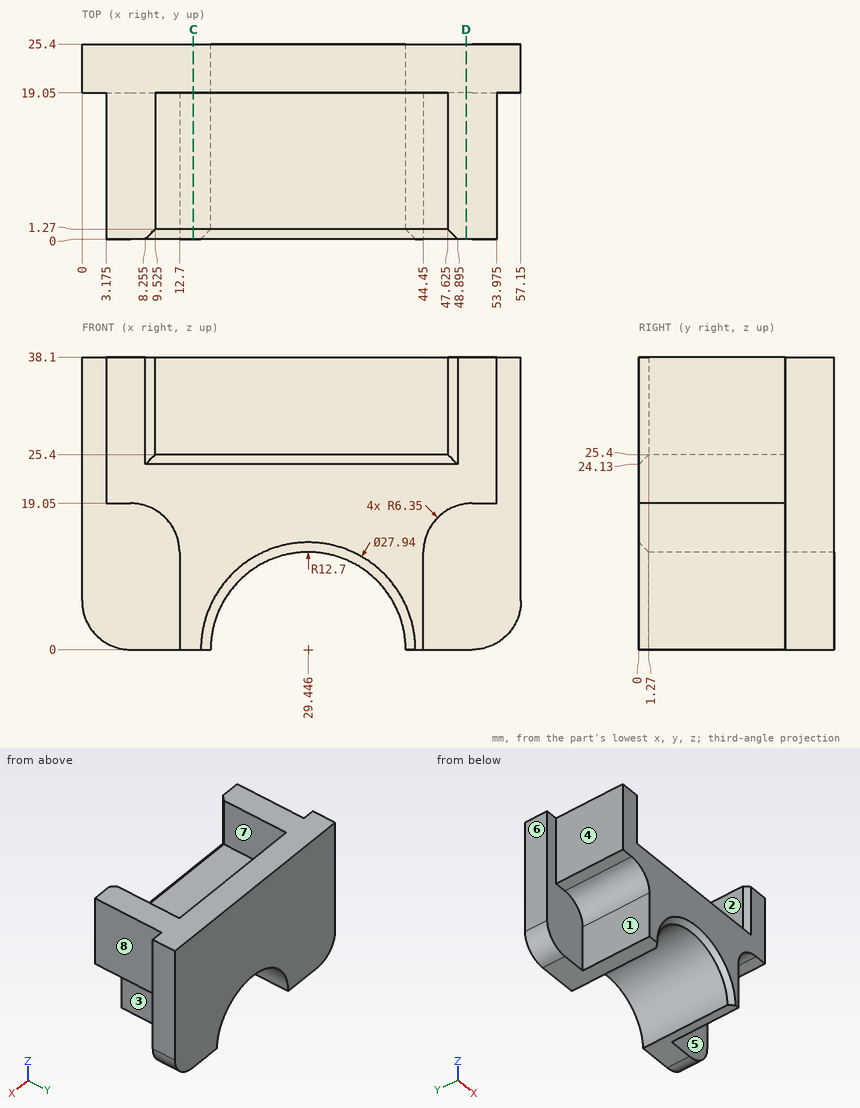
Verification items for this drawing (mm, ordinates from the low corner). A direction names the side the tool comes from. Round coordinates to 2 decimals unless told otherwise and drop trailing zeros. Order: outer loops, then holes, each group sorted by start corner. A loop starts at its lowest first (then second) coordinate and runs counter-clockwise, first axis right, second up. Notation, with made-up numbers: (59.25, -4) - (99.25, -4) arc R24 ccw to (99.25, 22) - close; hole circle Ø7 at (76.25, 38). An arc over 180 degrees is marked (long way). Use CSV: the item, a comma, the result in double quotes.
(1) Thickness scan on probe 1 along X at (y, z) = (19, 26) (1 decimal); probe 2 along Y at (x, z) = (47, 27); probe 3 along Z at (x, y) = (51, 7.5). Record the ranges inside material, lowest first. Write a range as from..to.
Entries:
probe 1,"3.2..9.5, 47.6..54"
probe 2,"19.05..25.4"
probe 3,"19.05..38.1"
(2) Section check D-D on x = 50. Record the boundary of the cut face in (y, z), and give its area (3 significant figures).
Entries:
outline,"(0, 19) - (19.05, 19) - (19.05, 0) - (25.4, 0) - (25.4, 38.1) - (0, 38.1) - close"
area,"606 mm^2"
(3) Access from +Z, -Z, +X, -X, +Y, -Y to the whole of each face (thin tool, end or side, straight path). Record for the marked faces 1, 2, 3 and 4.
Entries:
face 1,"-Z, -X, -Y"
face 2,"+Z, -Y"
face 3,"-Z, +X, -Y"
face 4,"+Z, -Z, -X, -Y"
(4) Section check C-C on x = 14.5. Record the boundary of the cut face in (y, z).
Entries:
outline,"(0, 0) - (25.4, 0) - (25.4, 38.1) - (19.05, 38.1) - (19.05, 25.4) - (1.27, 25.4) - (0, 24.13) - close"
(5) Mould release check, pull along X, two halves, no side actions. Record for the marked faces 5, 6, 7 and 8: released by +X, released by -X, zero draft, split by the parting line, or undercut.
Entries:
face 5,"zero draft"
face 6,"released by -X"
face 7,"undercut"
face 8,"released by +X"
(6) Gauge pin test, flat ends, axial feed: pin 1 Ø1 at (x, y) = (52.5, 10) entering from -Z; pin 2 Ø14 at (x, z) = (34, 30) entering from -Y; pin 3 Ø1 at (x, y) = (25, 18.5) entering from -Z; pin 4 Ø14 at (y, z) = (7.5, 4) entering from -X. Record the tip position at first contact, or that the pin passes through.
Entries:
pin 1,"z = 19.05"
pin 2,"y = 0"
pin 3,"z = 11.7"
pin 4,"x = 12.7"
